Autodesk Inventor part; units mm, degrees
ref_plane "YZ Plane" through (0, 0, 0) normal (1, 0, 0) x (0, 1, 0)
ref_plane "XZ Plane" through (0, 0, 0) normal (0, 1, 0) x (-1, 0, 0)
ref_plane "XY Plane" through (0, 0, 0) normal (0, 0, 1) x (1, 0, 0)
sketch "Sketch1" plane through (0, 0, 0) normal (0, 0, 1) x (1, 0, 0)
  line L0 (0, 0) -> (0, 6)
  line L1 (0, 6) -> (-4, 6)
  line L2 (-4, 6) -> (-4, -6)
  line L3 (-4, -6) -> (0, -6)
  line L4 (0, -6) -> (0, 6)
  line L5 (-2, 6) -> (-2, -6)
  line L6 (-2, 6) -> (-2, 3)
  circle A0 centre (-2, 3) radius 1.25
  line L7 (-2, -6) -> (-2, -3)
  circle A1 centre (-2, -3) radius 1.25
  line L8 (0, 6) -> (0, 14)
  line L9 (0, 14) -> (6, 14)
  line L10 (6, 14) -> (6, -22)
  line L11 (6, -22) -> (0, -22)
  line L12 (0, -22) -> (0, 14)
  dimension "d44" = 6
  dimension "d45" = 4
  dimension "d46" = 12
  dimension "d47" = 3
  dimension "d48" = 2.5
  dimension "d49" = 3
  dimension "d50" = 2.5
  dimension "d51" = 8
  dimension "d52" = 6
  dimension "d53" = 36
extrude "Extrusion8" add sketch "Sketch1" along normal mid plane 2 contours L4 L3 L5 A1 A0 L1 L0 | L5 A0 A1 L3 L2 L1
extrude "Extrusion9" add sketch "Sketch1" along normal mid plane 12 contours L0 L8 L9 L10 L11 L12 L4
fillet "Fillet1" radius 2 4 edges at (3, 14, 6) (3, 14, -6) (3, -22, 6) (3, -22, -6)
sketch "Sketch2" plane through (6, -20, -6) normal (1, 0, 0) x (0, 0, -1)
  point P0 (-6, 18)
properties part number "link7" material "Aluminum 6061"
Part model, mm, in its own coordinate system. A direction names the side the tool comes from. Round coordinates to 2 decimals unless told otherwise and drop trailing zeros. Order: outer loops, then holes, each group sorted by start corner. A loop starts at its lowest first (then second) coordinate and runs counter-clockwise, first axis right, second up. Notation, with made-up numbers: M 9.25,-37 L 38.25,-37 A22 cw 38.25,-31 Z; hole C -27.75,-24 d10. An arc over 180 degrees is marked long. Answer in a Markdown table with one row per item. Add a question column.
Q1. Cut at C-C on y = -5.5. Give the cut face in (x, z), and give its area (3 significant figures).
Q2. Cut at D-D on z = 2.5. Give the cut face in (x, y), and give its area (3 significant figures).
Q3. Cut at B-B on y = 3. Give the cut face in (x, z).
Q4. Cut at A-A on x = -2. Give the cut face in (y, z).
Q5. Wall check: L1, parallel to Y at x = -2, z = 0.5; L2, parallel to X at y = -3, z = 0.4; L3, parallel to X at y = -4, z = 5. Give the ranges that are in metal, low to high. Write a range as from..to.
Q6. Mould opens along Y. For faces 5 (the face through (-0.81, 2.62, -0.01)), 6 (the face through (3, -4, -6)), 7 (the face through (-0.81, -2.62, 0.01)), 8 (the face through (3, 14, 0)) say: +Y half, -Y half, draft (parallel to the pull), parting line (faces both ways), or undercut.
Q7. 3-axis set-ups, long thin cutter, end or side, ignore diameter. For faces 1 (the face through (-2, -6, 0)), 2 (the face through (-2, 0, -1)), 3 (the face through (-2, 6, 0)), 4 (the face through (-2, 0, 1)): which of +Z, -Z, +X, -X, +Y, -Y reach the whole face in a straight line?
Q8. Pin check, flat tips, straight feed: pin 1 (3 mm diameter, centred on x = -2.5, y = -2.5, fed in from +Z); pin 2 (2 mm diameter, centred on y = -16, z = 0.5, fed in from -X); pin 3 (0.6 mm diameter, centred on x = -2.5, z = -0.5, fed in from +Y). Stop position of each tip, or through.
Established:
| question | item | result |
|---|---|---|
| 1 | outline | M -4,-1 L 0,-1 L 0,-6 L 6,-6 L 6,6 L 0,6 L 0,1 L -4,1 Z |
| 1 | area | 80.0 mm2 |
| 2 | outline | M 0,-22 L 6,-22 L 6,14 L 0,14 Z |
| 2 | area | 216 mm2 |
| 3 | outline | M -4,-1 L -3.25,-1 L -3.25,1 L -4,1 Z; M -0.75,-1 L 0,-1 L 0,-6 L 6,-6 L 6,6 L 0,6 L 0,1 L -0.75,1 Z |
| 4 | outline | M -6,-1 L -4.25,-1 L -4.25,1 L -6,1 Z; M -1.75,-1 L 1.75,-1 L 1.75,1 L -1.75,1 Z; M 4.25,-1 L 6,-1 L 6,1 L 4.25,1 Z |
| 5 | L1 | y = -6..-4.25, -1.75..1.75, 4.25..6 |
| 5 | L2 | x = -4..-3.25, -0.75..6 |
| 5 | L3 | x = 0..6 |
| 6 | face 5 | undercut |
| 6 | face 6 | draft |
| 6 | face 7 | undercut |
| 6 | face 8 | +Y half |
| 7 | face 1 | +Z, -Z, -X, -Y |
| 7 | face 2 | -Z, -X, +Y, -Y |
| 7 | face 3 | +Z, -Z, -X, +Y |
| 7 | face 4 | +Z, -X, +Y, -Y |
| 8 | pin 1 | stops at z = 1 |
| 8 | pin 2 | stops at x = 0 |
| 8 | pin 3 | stops at y = 6 |
